from build123d import *

# Parameters (mm, degrees)
PAD_DEPTH       = 20
THICKNESS_T     = 2
SKETCH001_W     = 15
SKETCH001_H     = 2
PAD001_DEPTH    = 6
SKETCH002_R     = 1.4
POCKET_DEPTH    = 2.001
SKETCH003_W     = 15
SKETCH003_H     = 2
PAD002_DEPTH    = 6
SKETCH004_R     = 1.4
POCKET001_DEPTH = 22.001
SKETCH005_R     = 2.5
PAD003_DEPTH    = 7
SKETCH006_R     = 5
PAD004_DEPTH    = 5
SKETCH007_R     = 1.6
POCKET002_DEPTH = 22.001
SKETCH008_R     = 3.5
POCKET003_DEPTH = 2.8
SKETCH009_W     = 12.5
SKETCH009_H     = 4
POCKET004_DEPTH = 2


with BuildPart() as part:
    # Sketch → Pad (new body)
    with BuildSketch(Plane.XY):
        with BuildLine():
            Line((0, 37), (46, 37))
            ThreePointArc((49, 34), (48.1213203436, 36.1213203436), (46, 37))
            Line((49, 34), (49, 3))
            ThreePointArc((46, 0), (48.1213203436, 0.8786796564), (49, 3))
            Line((46, 0), (0, 0))
            ThreePointArc((-3, 3), (-2.1213203436, 0.8786796564), (0, 0))
            Line((-3, 3), (-3, 34))
            ThreePointArc((0, 37), (-2.1213203436, 36.1213203436), (-3, 34))
        make_face()
    extrude(amount=PAD_DEPTH)

    # Thickness
    thickness_openings = [part.faces().sort_by_distance(p)[0] for p in [
        (23, 18.5, 20),
    ]]
    offset(amount=THICKNESS_T, openings=thickness_openings, kind=Kind.INTERSECTION)

    # Sketch001 → Pad001 (new body)
    with BuildSketch(Plane(origin=(0, 39, 0), x_dir=(-1, 0, 0), z_dir=(0, 1, 0))):
        with Locations((-23, -1)):
            Rectangle(SKETCH001_W, SKETCH001_H)
    extrude(amount=PAD001_DEPTH)

    # Sketch002 → Pocket (cut, through all)
    with BuildSketch(Plane.XY):
        with Locations((23, 42)):
            Circle(SKETCH002_R)
    extrude(amount=-POCKET_DEPTH, mode=Mode.SUBTRACT)

    # Sketch003 → Pad002 (new body)
    with BuildSketch(Plane.XZ.offset(2)):
        with Locations((23, -1)):
            Rectangle(SKETCH003_W, SKETCH003_H)
    extrude(amount=PAD002_DEPTH)

    # Sketch004 → Pocket001 (cut, through all)
    with BuildSketch(Plane(origin=(0, 0, -2), x_dir=(1, 0, 0), z_dir=(0, 0, -1))):
        with Locations((23, 5)):
            Circle(SKETCH004_R)
    extrude(amount=-POCKET001_DEPTH, mode=Mode.SUBTRACT)

    # Sketch005 → Pad003 (new body)
    with BuildSketch(Plane(origin=(0, 0, -2), x_dir=(1, 0, 0), z_dir=(0, 0, -1))):
        with Locations((2, -18.5)):
            Circle(SKETCH005_R)
        with Locations((44, -18.5)):
            Circle(SKETCH005_R)
    extrude(amount=-PAD003_DEPTH)

    # Sketch006 → Pad004 (new body)
    with BuildSketch(Plane(origin=(0, 0, -2), x_dir=(1, 0, 0), z_dir=(0, 0, -1))):
        with Locations((2, -18.5)):
            Circle(SKETCH006_R)
        with Locations((44, -18.5)):
            Circle(SKETCH006_R)
    extrude(amount=-PAD004_DEPTH)

    # Sketch007 → Pocket002 (cut, through all)
    with BuildSketch(Plane(origin=(0, 0, -2), x_dir=(1, 0, 0), z_dir=(0, 0, -1))):
        with Locations((2, -18.5)):
            Circle(SKETCH007_R)
        with Locations((44, -18.5)):
            Circle(SKETCH007_R)
    extrude(amount=-POCKET002_DEPTH, mode=Mode.SUBTRACT)

    # Sketch008 → Pocket003 (cut)
    with BuildSketch(Plane(origin=(0, 0, -2), x_dir=(1, 0, 0), z_dir=(0, 0, -1))):
        with Locations((2, -18.5)):
            Circle(SKETCH008_R)
        with Locations((44, -18.5)):
            Circle(SKETCH008_R)
    extrude(amount=-POCKET003_DEPTH, mode=Mode.SUBTRACT)

    # Sketch009 → Pocket004 (cut)
    with BuildSketch(Plane.XZ.offset(2)):
        with Locations((11.75, 8)):
            Rectangle(SKETCH009_W, SKETCH009_H)
    extrude(amount=-POCKET004_DEPTH, mode=Mode.SUBTRACT)


solid = part.part
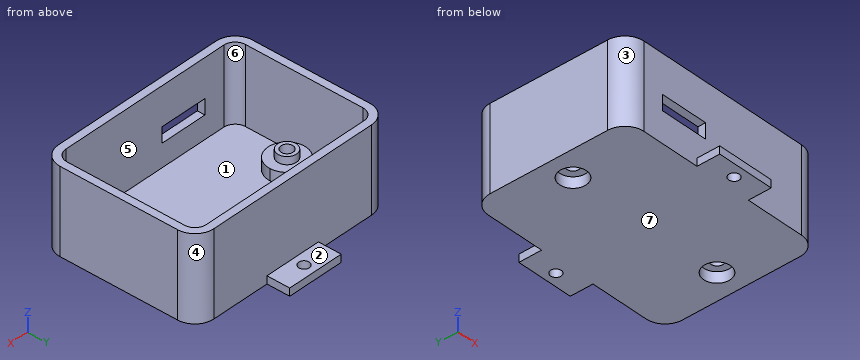
The model under review builds one solid part; all positions refer to its coordinate system, in mm. Face numbers are marked on the shaded views. A direction names the side the tool comes from. Coordinates: 2 decimals unless noted, no trailing zeros. Order: outer loops, then holes, each group sorted by start corner. A loop starts at its lowest first (then second) coordinate and runs counter-clockwise, first axis right, second up. Notation, with made-up numbers: (-38, -8) -> (2, -8) arc R19 ccw to (2, 16) -> close; hole circle Ø5 at (14, 27). An arc over 180 degrees is marked (long way). Answer in a Markdown table with one row per item.
(1) The part is to be moulded in two halves that separate along X. For the marked faces 4, 5, 6 and 7, say which applies: +X half, -X half, draft (parallel to the pull), parting line (faces both ways), or undercut.
Answers:
| item | result |
|---|---|
| face 4 | +X half |
| face 5 | undercut |
| face 6 | undercut |
| face 7 | draft |
(2) Consider section D-D (x = 33). Write out the cut boundary in (y, z), plus the area to 3 significant figures.
Answers:
| item | result |
|---|---|
| outline | (-2, -2) -> (39, -2) -> (39, 20) -> (37, 20) -> (37, 0) -> (0, 0) -> (0, 20) -> (-2, 20) -> close |
| area | 162 mm² |
(3) Insertion check: pin 1 (1.6 mm diameter, centred on y = -0.5, z = 7, fed in from +X); pin 2 (3 mm diameter, centred on x = 20, y = -4.5, fed in from +Z); pin 3 (6.5 mm diameter, centred on x = 44, y = 18.5, fed in from +Z); pin 4 (2.5 mm diameter, centred on x = 2, y = 18.5, fed in from +Z). Each pin has a flat end and moves straight along its axis. Give the tip position at first contact, or say it passes through.
Answers:
| item | result |
|---|---|
| pin 1 | x = 50.21 |
| pin 2 | z = 0 |
| pin 3 | z = 5 |
| pin 4 | through |
(4) Wall thickness on line 1 along Y through (x, z) = (2, 2.35); line 2 along X through (y, z) = (18.5, 4.1); line 3 along Y through (x, z) = (28.5, 18.5): over which ranges is each line inside the solid? List them lowest first.
Answers:
| item | result |
|---|---|
| line 1 | -2 to 0, 13.5 to 16.9, 20.1 to 23.5, 37 to 39 |
| line 2 | -5 to -3, -0.5 to 0.4, 3.6 to 4.5, 41.5 to 42.4, 45.6 to 46.5, 49 to 51 |
| line 3 | -2 to 0, 37 to 39 |
(5) Consider section B-B (x = 23). Write out the cut boundary in (y, z).
Answers:
| item | result |
|---|---|
| outline | (-8, -2) -> (-6.4, -2) -> (-6.4, 0) -> (-8, 0) -> close; (-3.6, -2) -> (40.6, -2) -> (40.6, 0) -> (39, 0) -> (39, 20) -> (37, 20) -> (37, 0) -> (0, 0) -> (0, 20) -> (-2, 20) -> (-2, 0) -> (-3.6, 0) -> close; (43.4, -2) -> (45, -2) -> (45, 0) -> (43.4, 0) -> close |
(6) Consider section C-C (y = -5). Write out the cut boundary in (x, z), plus the area to 3 significant figures.
Answers:
| item | result |
|---|---|
| outline | (15.5, -2) -> (21.6, -2) -> (21.6, 0) -> (15.5, 0) -> close; (24.4, -2) -> (30.5, -2) -> (30.5, 0) -> (24.4, 0) -> close |
| area | 24.4 mm² |
(7) Consider section A-A (z = 3.75). Write out the cut boundary in (x, y), plus the area to 3 significant figures.
Answers:
| item | result |
|---|---|
| outline | (-5, 3) arc R5 ccw to (0, -2) -> (46, -2) arc R5 ccw to (51, 3) -> (51, 34) arc R5 ccw to (46, 39) -> (0, 39) arc R5 ccw to (-5, 34) -> close; circle Ø5 at (2, 18.5); circle Ø5 at (44, 18.5); hole (-3, 3) arc R3 ccw to (0, 0) -> (46, 0) arc R3 ccw to (49, 3) -> (49, 34) arc R3 ccw to (46, 37) -> (0, 37) arc R3 ccw to (-3, 34) -> close; hole circle Ø3.2 at (2, 18.5); hole circle Ø3.2 at (44, 18.5) |
| area | 381 mm² |
(8) Machinability: for the marked faces 1, 2 and 3, which of the approach directions +Z, -Z, +X, -X, +Y, -Y give a long, thin tool a straight path to every point of the face, cutting with its end or side? Answer none if there is none.
Answers:
| item | result |
|---|---|
| face 1 | +Z |
| face 2 | +Z, +X, -X, +Y |
| face 3 | +Z, -Z, -X, -Y |
